from build123d import *

# Parameters (mm, degrees)
F1_DEPTH = 203.2
F2_W     = 88.9
F2_H     = 117.475


with BuildPart() as f1:
    # F0 (on Top) → F1 (new body)
    with BuildSketch(Plane.XY):
        with BuildLine():
            Line((1194.4176857661, 20132.1994861945), (1218.4865560082, 20537.8861257148))
            ThreePointArc((1218.4865560082, 20537.8861257148), (609.5108077566, 20564.9695495818), (0, 20574))
            Line((0, 20574), (0, 20167.6))
            ThreePointArc((0, 20167.6), (597.4710880973, 20158.7479288493), (1194.4176857661, 20132.1994861945))
        make_face()
    extrude(amount=F1_DEPTH)

    # F4: sweep along a path in F3
    with BuildLine(Plane.XY) as f4_path:
        ThreePointArc((1200.4349033266, 20233.6211460746), (600.4810180121, 20260.3033340325), (0, 20269.2))
    # F2 (on face) → F4 (sweep, cut)
    with BuildSketch(Plane(origin=(0, 0, 0), x_dir=(0.0592245823, 0.9982446839, 0), z_dir=(0.9982446839, -0.0592245823, 0))):
        with Locations((20313.65, 58.7375)):
            Rectangle(F2_W, F2_H)
    sweep(path=f4_path.line, mode=Mode.SUBTRACT)


solid = f1.part
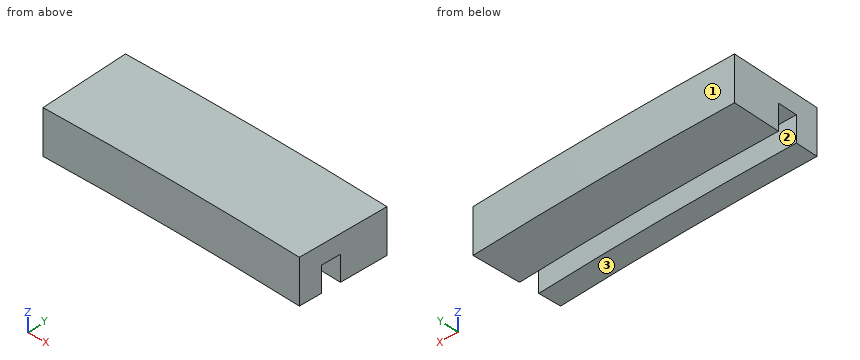
The model under review builds one solid part; all positions refer to its coordinate system, in mm. Face numbers are marked on the shaded views. Round coordinates to 2 decimals unless told otherwise and drop trailing zeros. Loops run counter-clockwise (first coordinate to the right, second up) from the corner with the lowest first, then second, coordinate; pieces in that order, holes last. Notation, with made-up numbers: (6.25, 73.25) -> (60.25, 73.25) arc R35 cw to (60.25, 109.25) -> close; hole circle Ø5 at (46.5, 45). An arc over 180 degrees is marked (long way). Return JSON: item names as keys, results as strings.
(1) Add section D-D on z = 160.5. Write out the cut boundary in (x, y), plus the area to 3 significant figures.
Solved:
{"outline": "(0, 20167.6) arc R20167.6 cw to (1194.42, 20132.2) -> (1218.49, 20537.89) arc R20574 ccw to (0, 20574) -> close", "area": "491,000 mm2"}
(2) Add section A-A on z = 51.5. Write out the cut boundary in (x, y), plus the area to 3 significant figures.
Solved:
{"outline": "(0, 20167.6) arc R20167.6 cw to (1194.42, 20132.2) -> (1200.43, 20233.62) arc R20269.2 ccw to (0, 20269.2) -> close; (0, 20358.1) arc R20358.1 cw to (1205.7, 20322.37) -> (1218.49, 20537.89) arc R20574 ccw to (0, 20574) -> close", "area": "384,000 mm2"}
(3) For pin 1 (1 mm diameter, centred on x = 456, y = 20499, fed in from -Z); pin 2 (6 mm diameter, centred on x = 208, y = 20342.5, fed in from -Z) (3 decimals), all flat-tipped, find the tip position at first contact; note any pin that passes through.
Solved:
{"pin 1": "z = 0", "pin 2": "z = 117.475"}
(4) The part is to be moulded in two halves that separate along Y. For the marked faces 1, 2 and 3, say which applies: released by +Y, released by -Y, zero draft, split by the parting line, or undercut.
Solved:
{"face 1": "released by +Y", "face 2": "undercut", "face 3": "zero draft"}
(5) Add section B-B on x = 285.5. Write out the cut boundary in (y, z) (3 decimals).
Solved:
{"outline": "(20165.579, 0) -> (20267.189, 0) -> (20267.189, 117.475) -> (20356.098, 117.475) -> (20356.098, 0) -> (20572.019, 0) -> (20572.019, 203.2) -> (20165.579, 203.2) -> close"}
(6) For line 1 (Y direction, x = 943.5, z = 51); line 2 (Z direction, x = 193, y = 20314) (3 decimals); line 3 (Y direction, x = 302, z = 23.5), list the stretches that pass through material, from the lowest coordinate up.
Solved:
{"line 1": "20145.52 to 20247.23, 20336.22 to 20552.35", "line 2": "117.475 to 203.2", "line 3": "20165.34 to 20266.95, 20355.86 to 20571.78"}
